from build123d import *

# Parameters (mm, degrees)
SKETCH1_W                = 43.18
SKETCH1_H                = 43.18
BOSS_EXTRUDE1_DEPTH      = 0.9
SKETCH2_R                = 1.7
CUT_EXTRUDE1_DEPTH       = 0.9
CIRPATTERN1_COUNT        = 4
BOSS_EXTRUDE2_DEPTH      = 0.9
BOSS_EXTRUDE2_DEPTH_BACK = 10
SKETCH5_W                = 24
SKETCH5_H                = 16
BOSS_EXTRUDE3_DEPTH      = 3


with BuildPart() as part:
    # Sketch1 → Boss-Extrude1 (new body)
    with BuildSketch(Plane(origin=(0, 0, 0), x_dir=(1, 0, 0), z_dir=(0, 1, 0))):
        with Locations((21.59, 21.59)):
            Rectangle(SKETCH1_W, SKETCH1_H)
    extrude(amount=BOSS_EXTRUDE1_DEPTH)

    # Sketch2 → Cut-Extrude1 (cut)
    with BuildSketch(Plane(origin=(0, 0.9, 0), x_dir=(1, 0, 0), z_dir=(0, 1, 0))):
        with Locations((2.54, 40.64)):
            Circle(SKETCH2_R)
    cut_extrude1 = extrude(amount=-CUT_EXTRUDE1_DEPTH, mode=Mode.SUBTRACT)

    # CirPattern1: Cut-Extrude1 ×4 about axis
    cirpattern1_axis = Axis((21.683217483, 0, -21.496782517), (0, 1, 0))
    for i in range(1, CIRPATTERN1_COUNT):
        add(cut_extrude1.rotate(cirpattern1_axis, i * 360 / CIRPATTERN1_COUNT), mode=Mode.SUBTRACT)

    # Sketch4 → Boss-Extrude2 (add, two sides)
    with BuildSketch(Plane.XY) as boss_extrude2_sk:
        with BuildLine():
            Line((27.49, 3.9), (34.18, 3.9))
            ThreePointArc((34.18, 3.9), (35.68, 2.4), (34.18, 0.9))
            Line((34.18, 0.9), (27.49, 0.9))
            ThreePointArc((27.49, 0.9), (25.99, 2.4), (27.49, 3.9))
        make_face()
        with BuildLine():
            Line((27.49, 2.8), (34.18, 2.8))
            ThreePointArc((34.18, 2.8), (34.58, 2.4), (34.18, 2))
            Line((34.18, 2), (27.49, 2))
            ThreePointArc((27.49, 2), (27.09, 2.4), (27.49, 2.8))
        make_face(mode=Mode.SUBTRACT)
    extrude(amount=BOSS_EXTRUDE2_DEPTH)
    extrude(boss_extrude2_sk.sketch, amount=-BOSS_EXTRUDE2_DEPTH_BACK)

    # Sketch5 → Boss-Extrude3 (add)
    with BuildSketch(Plane(origin=(0, 0.9, 0), x_dir=(1, 0, 0), z_dir=(0, 1, 0))):
        with Locations((22.747653051, 24.232550554)):
            Rectangle(SKETCH5_W, SKETCH5_H)
    extrude(amount=BOSS_EXTRUDE3_DEPTH)


solid = part.part
Can you work these out from the model? Positions are in its coordinate system, mm. A direction names the side the tool comes from. Coordinates: 2 decimals unless noted, no trailing zeros. Order: outer loops, then holes, each group sorted by start corner. A loop starts at its lowest first (then second) coordinate and runs counter-clockwise, first axis right, second up. Notation, with made-up numbers: (57.25, -35) - (82.25, -35) arc R32 cw to (82.25, -2) - close; hole circle Ø1 at (39.5, -36.75). An arc over 180 degrees is marked (long way). Answer as a JSON object with one key per item and string values. Group by question number.
Q1. Imagine slicing it at A-A (x = 2.54). Please give me the cut outline in (y, z), and give its area (3 significant figures).
Q2. Imagine slicing it at B-B (z = -3.5). Please give me the cut outline in (x, y).
Q3. Imagine slicing it at D-D (z = -40.64). Please give me the cut outline in (x, y), and give its area (3 significant figures).
Q4. On a 3-axis mill with a long thin cutter (end or side, diameter ignored), from which of +Z, -Z, +X, -X, +Y, -Y can I reach the whole of each face in a straight line? I mean faces 1 (the face through (23, 2, -16.233)), 2 (the face through (23, 2, -32.233)), 3 (the face through (31, 2.8, -4)), 4 (the face through (34.748, 2, -24)). Say none if no direction works.
Q5. I need wall thicknesses on line 1 (X direction, y = 0.25, z = -40.64); line 2 (Z direction, x = 2.54, y = 0.6); line 3 (X direction, y = 2.45, z = -2). Which ranges of each line are inside material? Lowest first, please. Write a range as from..to.
Q6. Imagine slicing it at C-C (x = 29.5). Please give me the cut outline in (y, z), and give its area (3 significant figures).
Q7. We'd pull the mould along X, two halves only. Please class faces 5 (the face through (4.11, 0.46, -39.99)), 6 (the face through (1.39, 0.46, -1.1)), 7 (the face through (31, 3, -10)), 8 (the face through (10.748, 2, -24)): +X half, -X half, draft (parallel to the pull), parting line (faces both ways), or undercut.
Q8. Will these pins go through, and if not, where does the flat tip stop? P1, Ø5.5, axis at x = 2.54, z = -2.35, coming from the +Y side; P2, Ø0.9, axis at y = 2.5, z = -21.5, coming from the +X side; P3, Ø2, axis at x = 12.5, y = 2.5, coming from the -Z side.
Determined:
{
 "1": {"outline": "(0, -43.18) - (0.9, -43.18) - (0.9, -42.34) - (0, -42.34) - close; (0, -38.94) - (0.9, -38.94) - (0.9, -4.05) - (0, -4.05) - close; (0, -0.65) - (0.9, -0.65) - (0.9, 0) - (0, 0) - close", "area": "32.7 mm2"},
 "2": {"outline": "(0, 0) - (1.28, 0) - (1.28, 0.9) - (0, 0.9) - close; (3.8, 0) - (39.57, 0) - (39.57, 0.9) - (34.18, 0.9) arc R1.5 ccw to (34.18, 3.9) - (27.49, 3.9) arc R1.5 ccw to (27.49, 0.9) - (3.8, 0.9) - close; (42.08, 0) - (43.18, 0) - (43.18, 0.9) - (42.08, 0.9) - close; hole (27.49, 2) - (34.18, 2) arc R0.4 ccw to (34.18, 2.8) - (27.49, 2.8) arc R0.4 ccw to start"},
 "3": {"outline": "(0, 0) - (0.84, 0) - (0.84, 0.9) - (0, 0.9) - close; (4.24, 0) - (39.13, 0) - (39.13, 0.9) - (4.24, 0.9) - close; (42.53, 0) - (43.18, 0) - (43.18, 0.9) - (42.53, 0.9) - close", "area": "32.7 mm2"},
 "4": {"face 1": "+X, -X, +Y", "face 2": "-Z, +X, -X, +Y", "face 3": "+Z", "face 4": "-Z, +X, +Y"},
 "5": {"line 1": "x = 0..0.84, 4.24..39.13, 42.53..43.18", "line 2": "z = -43.18..-42.34, -38.94..-4.05, -0.65..0", "line 3": "x = 25.99..27.09, 34.58..35.68"},
 "6": {"outline": "(0, -43.18) - (0.9, -43.18) - (0.9, -32.23) - (3.9, -32.23) - (3.9, -16.23) - (0.9, -16.23) - (0.9, -10) - (2, -10) - (2, 0.9) - (0.9, 0.9) - (0.9, 0) - (0, 0) - close; (2.8, -10) - (3.9, -10) - (3.9, 0.9) - (2.8, 0.9) - close", "area": "111 mm2"},
 "7": {"face 5": "undercut", "face 6": "undercut", "face 7": "draft", "face 8": "-X half"},
 "8": {"P1": "stops at y = 0.9", "P2": "stops at x = 34.75", "P3": "stops at z = -32.23"}
}
